Check sheet for the drawn part. Datum: minimum x, y, z corner. Units: mm. Give positions to 0.01 mm unless a question says otherwise; leave off trailing zeros. Order: outer loops, then holes, each group sorted by start corner. A loop starts at its lowest first (then second) coordinate and runs counter-clockwise, first axis right, second up. Notation, with made-up numbers: (-20, 71.5) - (9, 71.5) arc R17 ccw to (9, 95.5) - close; hole circle Ø11 at (13.25, 78). An arc over 180 degrees is marked (long way). Answer as a JSON object with one key per item and string values. Group by question number.
(1) Section check B-B (y = 2.5). Record the boundary of the cut face in (x, z), then the cut area to 3 significant figures.
(2) Section check A-A (z = 6.5). Record the boundary of the cut face in (x, y), then the cut area to 3 significant figures.
(3) Thickness scan on line 1 (Y direction, x = 0.1, z = 6); line 2 (Z direction, x = 0.15, y = 2.5). Record the ranges inside material, lowest first.
(4) Section check C-C (x = 0.2). Record the boundary of the cut face in (y, z), then the cut area to 3 significant figures.
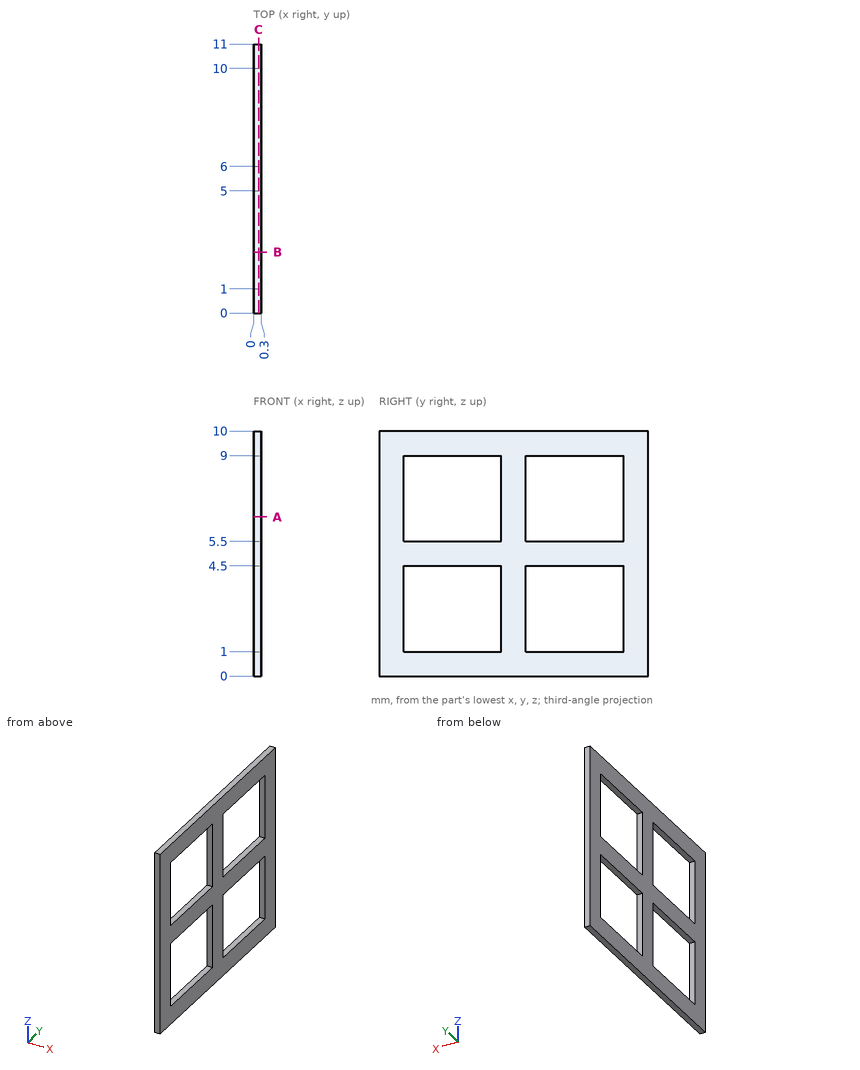
Solutions:
{
 "1": {"outline": "(0, 0) - (0.3, 0) - (0.3, 1) - (0, 1) - close; (0, 4.5) - (0.3, 4.5) - (0.3, 5.5) - (0, 5.5) - close; (0, 9) - (0.3, 9) - (0.3, 10) - (0, 10) - close", "area": "0.900 mm2"},
 "2": {"outline": "(0, 0) - (0.3, 0) - (0.3, 1) - (0, 1) - close; (0, 5) - (0.3, 5) - (0.3, 6) - (0, 6) - close; (0, 10) - (0.3, 10) - (0.3, 11) - (0, 11) - close", "area": "0.900 mm2"},
 "3": {"line 1": "y = 0 to 1, 5 to 6, 10 to 11", "line 2": "z = 0 to 1, 4.5 to 5.5, 9 to 10"},
 "4": {"outline": "(0, 0) - (11, 0) - (11, 10) - (0, 10) - close; hole (1, 1) - (5, 1) - (5, 4.5) - (1, 4.5) - close; hole (1, 5.5) - (5, 5.5) - (5, 9) - (1, 9) - close; hole (6, 1) - (10, 1) - (10, 4.5) - (6, 4.5) - close; hole (6, 5.5) - (10, 5.5) - (10, 9) - (6, 9) - close", "area": "54.0 mm2"}
}
